Read the model definition and answer for the solid it produces. Units are mm, in the model's axes. Face numbers are marked on the shaded views. A direction names the side the tool comes from. Coordinates: 2 decimals unless noted, no trailing zeros. Loops run counter-clockwise (first coordinate to the right, second up) from the corner with the lowest first, then second, coordinate; pieces in that order, holes last.
Q1. Section D-D (y = -25) is taken. Give the vertices of the cut face in (x, z), then the cut area to 3 significant figures.
Q2. Which of the six approach directions +Z, -Z, +X, -X, +Y, -Y give full straight-line access (tool end or side, diameter ignored) to the marked faces 1, 2 and 3?
Q3. Section C-C (x = 12) is taken. Give the vertices of the cut face in (y, z), then the cut area to 3 significant figures.
Q4. Section A-A (y = -6.5) is taken. Give the vertices of the cut face in (x, z).
Q5. Section B-B (y = -15) is taken. Give the vertices of the cut face in (x, z).
Q6. Straight lines are drawn through the part: line 1 (Y direction, x = 45, z = 1); line 2 (X direction, y = -17.5, z = 4.5); line 3 (Y direction, x = 39, z = 18). For each, find the intervals that lie inside material, in ascending order.
Q7. Flat-ended cylindrical pins translate along their axes: P1, Ø1.5, axis at x = 48, z = 58, coming from the -Y side; P2, Ø5, axis at y = -4, z = 64.5, coming from the +X side; P3, Ø6, axis at x = 62.5, y = -3.5, coming from the +Z side; P4, Ø9, axis at x = 45, y = -15, coming from the -Z side. Find the tip coordinate at first contact, or state that the pin passes through.
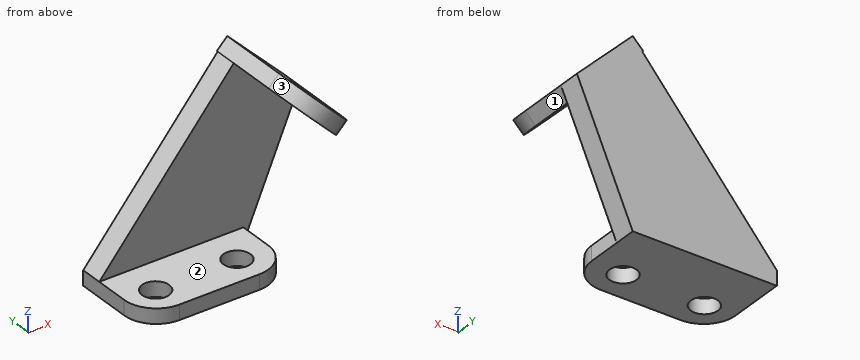
from build123d import *

# Parameters (mm, degrees)
F1_DEPTH = 9
F2_R     = 5.5
F3_DEPTH = 6
F5_R     = 7
F6_DEPTH = 6


with BuildPart() as f1:
    # F0 (on Front) → F1 (new body)
    with BuildSketch(Plane.XZ):
        Polygon((81.047416998, 52.686291501), (58.42, 75.313708499), (0, 6), (0, 0), (58.42, 0), align=None)
    extrude(amount=-F1_DEPTH)

    # F2 (on Top) → F3 (join)
    with BuildSketch(Plane.XY):
        with BuildLine():
            Line((58.42, 0), (0, 0))
            Line((0, 0), (0, -14))
            ThreePointArc((0, -14), (3.8076118446, -23.1923881554), (13, -27))
            Line((13, -27), (45.42, -27))
            ThreePointArc((45.42, -27), (54.6123881554, -23.1923881554), (58.42, -14))
            Line((58.42, -14), (58.42, 0))
        make_face()
        with Locations((12, -15)):
            Circle(F2_R, mode=Mode.SUBTRACT)
        with Locations((45, -15)):
            Circle(F2_R, mode=Mode.SUBTRACT)
    extrude(amount=F3_DEPTH)

    # F5 (on offset) → F6 (join)
    with BuildSketch(Plane(origin=(66.8668542495, 0, 66.8668542495), x_dir=(0, 1, 0), z_dir=(0.7071067812, 0, 0.7071067812))):
        with BuildLine():
            Line((9, -20.054344161), (9, 11.945655839))
            Line((9, 11.945655839), (-20, 11.945655839))
            ThreePointArc((-20, 11.945655839), (-36, -4.054344161), (-20, -20.054344161))
            Line((-20, -20.054344161), (9, -20.054344161))
        make_face()
        with Locations((-20, -4.054344161)):
            Circle(F5_R, mode=Mode.SUBTRACT)
    extrude(amount=-F6_DEPTH)


solid = f1.part
Numbers:
1. outline: (6.07, 0) - (52.35, 0) - (52.35, 6) - (6.07, 6) - close; (54.74, 70.5) - (62.03, 63.22) - (66.27, 67.46) - (58.99, 74.75) - close; (68.96, 56.29) - (76.24, 49.01) - (80.48, 53.25) - (73.2, 60.54) - close
1. area: 401 mm2
2. face 1: -Z, +X, -Y
2. face 2: +X, -X, -Y
2. face 3: -Y
3. outline: (-26.96, 0) - (-20.5, 0) - (-20.5, 6) - (-26.96, 6) - close; (-9.5, 0) - (9, 0) - (9, 20.24) - (0, 20.24) - (0, 6) - (-9.5, 6) - close
3. area: 278 mm2
4. outline: (0, 0) - (58.42, 0) - (58.42, 6) - (0, 6) - close; (54.18, 71.07) - (76.8, 48.44) - (81.05, 52.69) - (58.42, 75.31) - close
5. outline: (0.04, 0) - (6.5, 0) - (6.5, 6) - (0.04, 6) - close; (17.5, 0) - (39.5, 0) - (39.5, 6) - (17.5, 6) - close; (50.5, 0) - (58.38, 0) - (58.38, 6) - (50.5, 6) - close; (54.18, 71.07) - (62.03, 63.22) - (66.27, 67.46) - (58.42, 75.31) - close; (68.96, 56.29) - (76.8, 48.44) - (81.05, 52.69) - (73.2, 60.54) - close
6. line 1: y = -27 to -20.5, -9.5 to 9
6. line 2: x = 0.48 to 7.1, 16.9 to 40.1, 49.9 to 57.94
6. line 3: y = 0 to 9
7. P1: stops at y = 0
7. P2: stops at x = 71.73
7. P3: stops at z = 74.23
7. P4: passes through
